Design review of the part built by this model. Coordinates are the model's own, in mm. A direction names the side the tool comes from. Give positions to 0.01 mm unless a question says otherwise; leave off trailing zeros. Loops run counter-clockwise (first coordinate to the right, second up) from the corner with the lowest first, then second, coordinate; pieces in that order, holes last. Notation, with made-up numbers: (34, 81) - (70, 81) arc R15 cw to (70, 102) - close; hole circle Ø2 at (67.5, -38.5). An arc over 180 degrees is marked (long way). Put each result on its own line as item: value. Start each with the question number.
```python
from build123d import *

# Parameters (mm, degrees)
F1_DEPTH = 48.26
F2_DEPTH = 28.448
F3_DEPTH = 17.272
F4_W     = 25.4
F4_H     = 10.16
F5_DEPTH = 25.4
F6_R     = 6.35
F7_DEPTH = 46.482


with BuildPart() as f1:
    # F0 (on Top) → F1 (new body)
    with BuildSketch(Plane.XY):
        Polygon((0, 12.7), (0, 0), (30.48, 0), (30.48, 12.7), (30.48, 48.26), (30.48, 60.96), (0, 60.96), (0, 48.26), (10.16, 48.26), (10.16, 12.7), align=None)
    extrude(amount=F1_DEPTH)

    # F0 (on Top) → F2 (join)
    with BuildSketch(Plane.XY):
        Polygon((30.48, 48.26), (30.48, 12.7), (88.584137, 12.7), (100.076, 19.33483), (100.076, 41.62517), (88.584137, 48.26), align=None)
    extrude(amount=F2_DEPTH)

    # F0 (on Top) → F3 (join)
    with BuildSketch(Plane.XY):
        Polygon((100.076, 41.62517), (100.076, 19.33483), (119.38, 30.48), align=None)
    extrude(amount=F3_DEPTH)

    # F4 (on face) → F5 (cut)
    with BuildSketch(Plane(origin=(10.16, 0, 0), x_dir=(0, -1, 0), z_dir=(-1, 0, 0))):
        with Locations((-30.48, 43.18)):
            Rectangle(F4_W, F4_H)
    extrude(amount=-F5_DEPTH, mode=Mode.SUBTRACT)

    # F6 (on face) → F7 (cut)
    with BuildSketch(Plane.XZ.offset(-12.7)):
        with Locations((65.532, 14.224)):
            Circle(F6_R)
    extrude(amount=-F7_DEPTH, mode=Mode.SUBTRACT)


solid = f1.part
```
Item 1: Consider section B-B (y = 39). State the section outline as (x, z) points, plus the area to 3 significant figures.
Item 2: Consider section D-D (x = 69). State the section outline as (y, z) points.
Item 3: Consider section A-A (z = 42.5). State the section outline as (x, y) points, plus the area to 3 significant figures.
Item 4: Consider section C-C (z = 5.5). State the section outline as (x, y) points, plus the area to 3 significant figures.
Item 5: For L1, parallel to Z at x = 77.5, y = 19; L2, parallel to Z at x = 101, y = 30; L3, parallel to X at y = 3.5, z = 25, list the stretches that pass through material, from the lowest coordinate up. Write a range as from..to.
Item 6: Machinability: for faces 1 (the flat face through (100.076, 30, 23)), 2 (the flat face through (59.9, 48.26, 10.9)), 3 (the flat face through (20, 31, 38.1)), which of the approach directions +Z, -Z, +X, -X, +Y, -Y give a long, thin tool a straight path to every point of the face, cutting with its end or side? Answer none if there is none.
Item 7: For P1, Ø14, axis at x = 53, z = 17, coming from the -Y side; P2, Ø6, axis at x = 54, z = 21, coming from the +Y side; P3, Ø4, axis at y = 26.5, z = 28, coming from the +X side, all flat-tipped, find the tip position at first contact; note any pin that passes through.
Item 8: Mouldability with a two-part tool opening along Y and no side actions: class faces 4 (the flat face through (20, 43.18, 43)), 5 (the cylindrical face through (68.946, 30.231, 19.578)), 6 (the flat face through (15, 60.96, 24)) as pulls with the +Y half, pulls with the -Y half, needs draft (parallel to the pull), parting line crosses it, or undercut.
Geometry says:
1. outline: (10.16, 0) - (104.62, 0) - (104.62, 17.27) - (100.08, 17.27) - (100.08, 28.45) - (30.48, 28.45) - (30.48, 38.1) - (10.16, 38.1) - close; hole circle Ø12.7 at (65.53, 14.22)
1. area: 2,710 mm2
2. outline: (12.7, 0) - (48.26, 0) - (48.26, 8.9) - (12.7, 8.9) - close; (12.7, 19.54) - (48.26, 19.54) - (48.26, 28.45) - (12.7, 28.45) - close
3. outline: (0, 0) - (30.48, 0) - (30.48, 17.78) - (10.16, 17.78) - (10.16, 12.7) - (0, 12.7) - close; (0, 48.26) - (10.16, 48.26) - (10.16, 43.18) - (30.48, 43.18) - (30.48, 60.96) - (0, 60.96) - close
3. area: 981 mm2
4. outline: (0, 0) - (30.48, 0) - (30.48, 12.7) - (88.58, 12.7) - (119.38, 30.48) - (88.58, 48.26) - (30.48, 48.26) - (30.48, 60.96) - (0, 60.96) - (0, 48.26) - (10.16, 48.26) - (10.16, 12.7) - (0, 12.7) - close
4. area: 4,110 mm2
5. L1: z = 0..28.45
5. L2: z = 0..17.27
5. L3: x = 0..30.48
6. face 1: +Z, +X, +Y, -Y
6. face 2: +Z, -Z, +X, +Y
6. face 3: +Z, +X, -X
7. P1: stops at y = 12.7
7. P2: stops at y = 48.26
7. P3: stops at x = 100.08
8. face 4: undercut
8. face 5: needs draft
8. face 6: pulls with the +Y half
